Verification items for the finished model (mm, model axes). Round coordinates to 2 decimals unless told otherwise and drop trailing zeros. Write each loop counter-clockwise with the first axis right and the second up, starting at its lowest first coordinate (ties: lowest second). Pieces come first, ordered by that corner, then holes. Notation, with made-up numbers: (54, 65) - (99, 65) arc R18 cw to (99, 70) - close; hole circle Ø11 at (16.5, 1). An arc over 180 degrees is marked (long way). Answer as a JSON object with one key per item and string values.
```python
from build123d import *

# Parameters (mm, degrees)
SKETCH_1_R      = 1.6
EXTRUDE_1_DEPTH = 2
FILLET_1_R      = 4


with BuildPart() as part:
    # ｽｹｯﾁ1 → ﾎﾞｽ - 押し出し1 (new body)
    with BuildSketch(Plane.XY):
        Polygon((40.25, 37.5), (-30.25, 37.5), (-30.25, 28.5), (-40.25, 28.5), (-40.25, -28.5), (-30.25, -28.5), (-30.25, -37.5), (40.25, -37.5), align=None)
        with Locations((-24.75, -30)):
            Circle(SKETCH_1_R, mode=Mode.SUBTRACT)
        with Locations((35.25, -30)):
            Circle(SKETCH_1_R, mode=Mode.SUBTRACT)
        with Locations((-24.75, 30)):
            Circle(SKETCH_1_R, mode=Mode.SUBTRACT)
        with Locations((35.25, 30)):
            Circle(SKETCH_1_R, mode=Mode.SUBTRACT)
    extrude(amount=EXTRUDE_1_DEPTH)

    # ﾌｨﾚｯﾄ1
    fillet_1_edges = [part.edges().sort_by_distance(p)[0] for p in [
        (-30.25, -28.5, 1),
        (-30.25, 28.5, 1),
        (40.25, 37.5, 1),
        (40.25, -37.5, 1),
    ]]
    fillet(fillet_1_edges, radius=FILLET_1_R)


solid = part.part
```
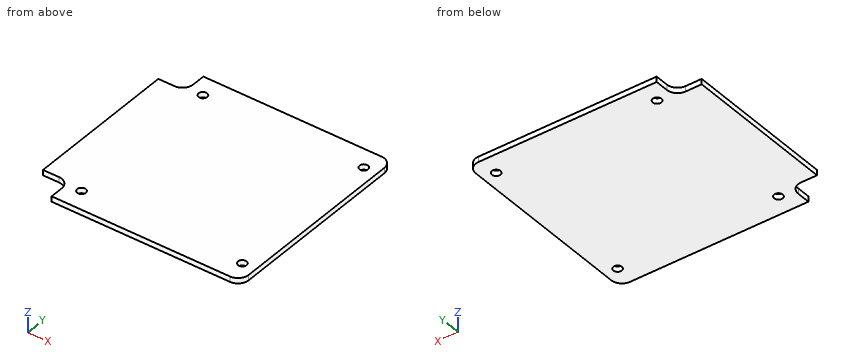
Q1. Section check A-A, the plane x = 35.25. Record the cut outline in (y, z).
Geometry check:
{"outline": "(-37.5, 0) - (-31.6, 0) - (-31.6, 2) - (-37.5, 2) - close; (-28.4, 0) - (28.4, 0) - (28.4, 2) - (-28.4, 2) - close; (31.6, 0) - (37.5, 0) - (37.5, 2) - (31.6, 2) - close"}
Q2. Gauge pin test, flat ends, axial feed: P1, Ø1, axis at y = 36, z = 1, coming from the -X side; P2, Ø0.6, axis at x = -38.5, z = 1.5, coming from the +Y side. Record the tip position at first contact, or that the pin passes through.
Geometry check:
{"P1": "stops at x = -30.25", "P2": "stops at y = 28.5"}
Q3. Section check B-B, the plane y = -30. Record the cut outline in (x, z).
Geometry check:
{"outline": "(-31.13, 0) - (-26.35, 0) - (-26.35, 2) - (-31.13, 2) - close; (-23.15, 0) - (33.65, 0) - (33.65, 2) - (-23.15, 2) - close; (36.85, 0) - (40.25, 0) - (40.25, 2) - (36.85, 2) - close"}
Q4. Material ranges on line 1 along Y through (x, z) = (-24.75, 1.1); line 2 along Y through (x, z) = (34, 1.7); line 3 along Y through (x, z) = (-36.5, 1.8), recorded low to high. Write a range as [from, to].
Geometry check:
{"line 1": "y = [-37.5, -31.6], [-28.4, 28.4], [31.6, 37.5]", "line 2": "y = [-37.5, -31], [-29, 29], [31, 37.5]", "line 3": "y = [-28.5, 28.5]"}
Q5. Section check C-C, the plane z = 0.9. Record the cut outline in (x, y).
Geometry check:
{"outline": "(-40.25, -28.5) - (-34.25, -28.5) arc R4 cw to (-30.25, -32.5) - (-30.25, -37.5) - (36.25, -37.5) arc R4 ccw to (40.25, -33.5) - (40.25, 33.5) arc R4 ccw to (36.25, 37.5) - (-30.25, 37.5) - (-30.25, 32.5) arc R4 cw to (-34.25, 28.5) - (-40.25, 28.5) - close; hole circle Ø3.2 at (-24.75, -30); hole circle Ø3.2 at (-24.75, 30); hole circle Ø3.2 at (35.25, -30); hole circle Ø3.2 at (35.25, 30)"}
